Input: part model. Units: mm. Frame: model coordinates. Face numbers are marked on the shaded views. A direction names the side the tool comes from. Coordinates: 2 decimals unless noted, no trailing zeros. Loops run counter-clockwise (first coordinate to the right, second up) from the corner with the lowest first, then second, coordinate; pieces in that order, holes last. Notation, with made-up numbers: (-6.5, 20.25) - (5.5, 20.25) arc R16 cw to (5.5, 32.25) - close; hole circle Ø10 at (-27.75, 27.5). An arc over 180 degrees is marked (long way). Use a Markdown table: item, result. Add a question column.
1. Draft query along Y for the marked faces 4, 5, 6 and 7. Return one class per face: released by +Y, released by -Y, zero draft, split by the parting line, or undercut.
2. Ray query, L1, parallel to X at y = -4.5, z = 17.5; L2, parallel to Y at x = -4.5, z = 46; L3, parallel to Y at x = 14, z = 46.5. Return the intervals inside material, ascending. Write a range as [from, to].
3. Access query for the marked faces 1, 2 and 3. Directions: +Z, -Z, +X, -X, +Y, -Y. A direction counts if a zero-diameter tool reaches every point of the face in a straight line with its end or side. Return the directions, or none.
4. Contact query for flat-ended pins moving along their axis: P1, Ø3, axis at x = -39.5, y = -35.5, coming from the -Z side; P2, Ø12.5, axis at x = -9.5, z = 43.5, coming from the -Y side; P3, Ø13.5, axis at y = 0, z = 33, coming from the -X side; P4, Ø13.5, axis at y = -4, z = 13.5, coming from the +X side. Output: stop coordinate, or through.
5. Section query C-C on y = 0. Return the cut outline in (x, z), then the cut area to 3 significant figures.
6. Section query B-B on x = 0. Return the cut outline in (y, z).
7. Section query D-D on y = -44. Return the cut outline in (x, z) (3 decimals), then the cut area to 3 significant figures.
8. Section query A-A on y = -36.5. Return the cut outline in (x, z), then the cut area to 3 significant figures.
```python
from build123d import *

# Parameters (mm, degrees)
SKETCH_1_W          = 50
SKETCH_1_H          = 10
EXTRUDE_1_DEPTH     = 50
EXTRUDE_3_DEPTH     = 25
SKETCH_5_R          = 5
CUT_EXTRUDE_2_DEPTH = 106.59356041


with BuildPart() as part:
    # 草图1 → 凸台-拉伸1 (new body)
    with BuildSketch(Plane.XY):
        Rectangle(SKETCH_1_W, SKETCH_1_H)
    extrude(amount=EXTRUDE_1_DEPTH)

    # 草图4 → 凸台-拉伸3 (add)
    with BuildSketch(Plane(origin=(0, 0, 0), x_dir=(-1, 0, 0), z_dir=(0, 0, -1))):
        with BuildLine():
            Line((-25, -5), (25, -5))
            Line((25, -5), (25, -11.698729811))
            ThreePointArc((25, -11.698729811), (43.301270189, -30), (50, -55))
            Line((50, -55), (46, -55))
            ThreePointArc((46, -55), (0, -9), (-46, -55))
            Line((-46, -55), (-50, -55))
            ThreePointArc((-50, -55), (-43.301270189, -30), (-25, -11.698729811))
            Line((-25, -11.698729811), (-25, -5))
        make_face()
    extrude(amount=-EXTRUDE_3_DEPTH)

    # 草图5 → 切除-拉伸2 (cut, through all)
    with BuildSketch(Plane(origin=(25, 0, 0), x_dir=(0, 0, -1), z_dir=(1, 0, 0))):
        with Locations((-50, 0)):
            Circle(SKETCH_5_R)
    extrude(amount=-CUT_EXTRUDE_2_DEPTH, mode=Mode.SUBTRACT)


solid = part.part
```
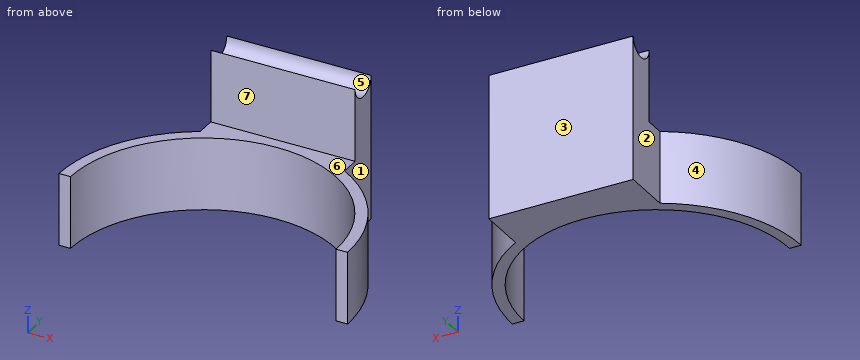
Resolved:
| question | item | result |
|---|---|---|
| 1 | face 4 | released by +Y |
| 1 | face 5 | undercut |
| 1 | face 6 | zero draft |
| 1 | face 7 | released by -Y |
| 2 | L1 | [-25, 25] |
| 2 | L2 | [-5, -3], [3, 5] |
| 2 | L3 | [-5, -3.57], [3.57, 5] |
| 3 | face 1 | +Z, -Z, +X, +Y |
| 3 | face 2 | +Z, -Z, -X, +Y |
| 3 | face 3 | +Z, -Z, +X, -X, +Y |
| 4 | P1 | through |
| 4 | P2 | y = -5 |
| 4 | P3 | x = -25 |
| 4 | P4 | x = 25 |
| 5 | outline | (-25, 0) - (25, 0) - (25, 45) - (-25, 45) - close |
| 5 | area | 2,250 mm² |
| 6 | outline | (-9, 0) - (5, 0) - (5, 50) arc R5 cw to (-5, 50) - (-5, 25) - (-9, 25) - close |
| 7 | outline | (-48.775, 0) - (-44.665, 0) - (-44.665, 25) - (-48.775, 25) - close; (44.665, 0) - (48.775, 0) - (48.775, 25) - (44.665, 25) - close |
| 7 | area | 205 mm² |
| 8 | outline | (-46.45, 0) - (-42.12, 0) - (-42.12, 25) - (-46.45, 25) - close; (42.12, 0) - (46.45, 0) - (46.45, 25) - (42.12, 25) - close |
| 8 | area | 217 mm² |
